The listing builds one solid part. Answer for the finished solid, in the listing's coordinates (mm). Face numbers are marked on the shaded views. A direction names the side the tool comes from. Coordinates: 2 decimals unless noted, no trailing zeros. Loops run counter-clockwise (first coordinate to the right, second up) from the corner with the lowest first, then second, coordinate; pieces in that order, holes last. Notation, with made-up numbers: M 2,-27.5 L 51,-27.5 A18 cw 51,-8.5 Z; hole C 0,-1 d6. An arc over 180 degrees is marked long. Answer as a JSON object with one key per item and string values. Group by question number.
1. A cutting plane is placed at B-B on x = -224. Give the vertices of the cut face in (y, z), and give its area (3 significant figures).
2. A cutting plane is placed at A-A on y = 261.5. Give the vertices of the cut face in (x, z).
3. Given pin 1 (9.5 mm diameter, centred on y = 180.5, z = 70.5, fed in from -X); pin 2 (6 mm diameter, centred on y = 60.5, z = 75, fed in from +X); pin 3 (7.5 mm diameter, centred on y = 110.5, z = 70.5, fed in from -X); pin 4 (9 mm diameter, centred on x = -380, z = 141.75, fed in from -Y), each flat-ended and moving along its own axis, determine where each tip first touches the part or whether it passes through.
4. For the marked faces 1 and 2, determine the directions among +Z, -Z, +X, -X, +Y, -Y from which every point of the face is accessible in a straight line to the end or side of a thin tool.
5. A cutting plane is placed at C-C on z = 91.5. Give the vertices of the cut face in (x, y).
6. Straight lines are drawn through the part: L1, parallel to Z at x = -380, y = 16; L2, parallel to X at y = 19, z = 79.25; L3, parallel to Z at x = -440, y = 180.5. For each, find the intervals that lie inside material, in ascending order.
7. A cutting plane is placed at D-D on y = 125. Give the vertices of the cut face in (x, z), and give its area (3 significant figures).
Autodesk Inventor part; units mm, degrees
ref_plane "YZ Plane" through (0, 0, 0) normal (1, 0, 0) x (0, 1, 0)
ref_plane "XZ Plane" through (0, 0, 0) normal (0, 1, 0) x (-1, 0, 0)
ref_plane "XY Plane" through (0, 0, 0) normal (0, 0, 1) x (1, 0, 0)
sketch "Sketch5" plane through (0, 0, 0) normal (0, 1, 0) x (-1, 0, 0)
  line L0 (452.5, 48) -> (452.5, 173)
  line L1 (117.5, 98) -> (117.5, 48)
  line L2 (117.5, 48) -> (452.5, 48)
  line L3 (67.5, 173) -> (67.5, 98)
  line L4 (67.5, 98) -> (117.5, 98)
  line L5 (67.5, 173) -> (452.5, 173)
  dimension "d8" = 125
  dimension "d13" = 385
  dimension "d18" = 50
  dimension "d42" = 50
extrude "Extrusion5" add sketch "Sketch5" along normal blind 291
sketch "Sketch6" plane through (0, 291, 0) normal (0, 1, 0) x (1, 0, 0)
  line L0 (-452.5, -173) -> (-67.5, -173)
  line L1 (-117.5, -48) -> (-452.5, -48)
  circle A0 centre (-140, -141.75) radius 6
  circle A1 centre (-140, -79.25) radius 6
  circle A2 centre (-260, -141.75) radius 6
  circle A3 centre (-260, -79.25) radius 6
  circle A4 centre (-380, -141.75) radius 6
  circle A5 centre (-380, -79.25) radius 6
  line L2 (-452.5, -48) -> (-452.5, -173)
  line L3 (-67.5, -173) -> (-67.5, -98)
  point P0 (0, 0)
  point P1 (-260, -173)
  dimension "d19" = 12
  dimension "d20" = 120
  dimension "d21" = 385
  dimension "d22" = 125
  dimension "d23" = 120
  dimension "d24" = 62.5
  dimension "d25" = 31.25
  dimension "d26" = 31.25
  dimension "d41" = 72.5
  dimension "d61" = 72.5
  dimension "d62" = 192.5
hole "Hole1" at (-140, 291, 141.75) at (-260, 291, 141.75) at (-380, 291, 141.75) at (-380, 291, 79.25) at (-260, 291, 79.25) at (-140, 291, 79.25) direction (0, -1, 0) diameter 10.106 depth 35 tip angle 118
sketch "Sketch7" plane through (0, 0, 0) normal (0, -1, 0) x (1, 0, 0)
  circle A0 centre (-380, 141.75) radius 5.053
  circle A1 centre (-380, 79.25) radius 5.053
  circle A2 centre (-260, 141.75) radius 5.053
  circle A3 centre (-260, 79.25) radius 5.053
  circle A4 centre (-140, 141.75) radius 5.053
  circle A5 centre (-140, 79.25) radius 5.053
  circle A6 centre (-140, 141.75) radius 5.053
  circle A7 centre (-140, 79.25) radius 5.053
  circle A8 centre (-260, 79.25) radius 5.053
  circle A9 centre (-260, 141.75) radius 5.053
  circle A10 centre (-380, 141.75) radius 5.053
  circle A11 centre (-380, 79.25) radius 5.053
  point P0 (0, 0)
hole "Hole2" at (-380, 0, 141.75) at (-380, 0, 79.25) at (-260, 0, 79.25) at (-260, 0, 141.75) at (-140, 0, 141.75) at (-140, 0, 79.25) direction (0, 1, 0) diameter 10.106 depth 35 tip angle 118
chamfer "Chamfer1" distance 5 angle 45 2 edges at (-67.5, 145.5, 98) (-117.5, 145.5, 48)
sketch "Sketch8" plane through (0, 291, 0) normal (0, 1, 0) x (1, 0, 0)
  line L0 (-182.5, -141.75) -> (-207.5, -141.75) construction
  line L1 (-182.5, -135.75) -> (-207.5, -135.75)
  line L2 (-207.5, -147.75) -> (-182.5, -147.75)
  arc A0 (-182.5, -147.75) -> (-182.5, -135.75) centre (-182.5, -141.75) ccw
  arc A1 (-207.5, -135.75) -> (-207.5, -147.75) centre (-207.5, -141.75) ccw
  line L3 (-427.5, -141.75) -> (-452.5, -141.75) construction
  line L4 (-427.5, -135.75) -> (-452.5, -135.75)
  line L5 (-452.5, -147.75) -> (-427.5, -147.75)
  arc A2 (-427.5, -147.75) -> (-427.5, -135.75) centre (-427.5, -141.75) ccw
  arc A3 (-452.5, -135.75) -> (-452.5, -147.75) centre (-452.5, -141.75) ccw
  line L6 (-452.5, -48) -> (-452.5, -173)
  circle A4 centre (-260, -141.75) radius 5.053
  point P0 (0, 0)
  point P1 (-440, -141.75)
  point P2 (-195, -141.75)
  point P3 (-440, -141.75)
  point P4 (-195, -147.75)
  point P5 (-195, -141.75)
  dimension "d46" = 12
  dimension "d47" = 12
  dimension "d48" = 25
  dimension "d49" = 25
  dimension "d58" = 12.5
  dimension "d60" = 257.5
extrude "Extrusion6" cut sketch "Sketch8" against normal blind 5 contours A0 L2 A1 L1 | A2 L5 L6 L4 | L6 A3
sketch "Sketch9" plane through (0, 0, 0) normal (0, -1, 0) x (1, 0, 0)
  line L0 (-452.5, 141.75) -> (-427.5, 141.75) construction
  line L1 (-452.5, 135.75) -> (-427.5, 135.75)
  line L2 (-427.5, 147.75) -> (-452.5, 147.75)
  arc A0 (-452.5, 147.75) -> (-452.5, 135.75) centre (-452.5, 141.75) ccw
  arc A1 (-427.5, 135.75) -> (-427.5, 147.75) centre (-427.5, 141.75) ccw
  line L3 (-207.5, 141.75) -> (-182.5, 141.75) construction
  line L4 (-207.5, 135.75) -> (-182.5, 135.75)
  line L5 (-182.5, 147.75) -> (-207.5, 147.75)
  arc A2 (-207.5, 147.75) -> (-207.5, 135.75) centre (-207.5, 141.75) ccw
  arc A3 (-182.5, 135.75) -> (-182.5, 147.75) centre (-182.5, 141.75) ccw
  arc A4 (-427.5, 135.75) -> (-427.5, 147.75) centre (-427.5, 141.75) ccw
  arc A5 (-207.5, 147.75) -> (-207.5, 135.75) centre (-207.5, 141.75) ccw
  arc A6 (-182.5, 135.75) -> (-182.5, 147.75) centre (-182.5, 141.75) ccw
  line L6 (-452.5, 48) -> (-452.5, 173)
  point P0 (0, 0)
  point P1 (-440, 141.75)
  point P2 (-195, 141.75)
  dimension "d76" = 25
  dimension "d77" = 25
  dimension "d78" = 12.5
extrude "Extrusion7" cut sketch "Sketch9" against normal blind 5
sketch "Sketch10" plane through (-452.5, 0, 48) normal (0, 0, -1) x (-1, 0, 0)
  line L0 (0, 0) -> (0, 291)
  line L1 (-330, 291) -> (0, 291)
  circle A0 centre (-295, 145.5) radius 5
  circle A1 centre (-165, 145.5) radius 5
  circle A2 centre (-35, 145.5) radius 5
  point P0 (-452.5, 0)
  point P1 (0, 145.5)
  point P2 (-165, 291)
  dimension "d63" = 130
  dimension "d64" = 130
  dimension "d65" = 10
hole "Hole3" at (-157.5, 145.5, 48) at (-287.5, 145.5, 48) at (-417.5, 145.5, 48) direction (0, 0, 1) diameter 8.376 depth 25 tip angle 118
chamfer "Chamfer2" distance 0.5 angle 45 14 edges at (-195, 291, 147.75) (-213.5, 291, 141.75) (-195, 291, 135.75) (-176.5, 291, 141.75) (-440, 291, 147.75) (-440, 291, 135.75) (-421.5, 291, 141.75) (-213.5, 0, 141.75) (-195, 0, 147.75) (-176.5, 0, 141.75) (-195, 0, 135.75) (-440, 0, 147.75) (-421.5, 0, 141.75) (-440, 0, 135.75)
chamfer "Chamfer3" distance 2 angle 45 3 edges at (-67.5, 145.5, 173) (-452.5, 145.5, 173) (-452.5, 145.5, 48)
sketch "Sketch11" plane through (-450.5, 0, 173) normal (0, 0, 1) x (1, 0, 0)
  circle A0 centre (226.5, 145.5) radius 7.5
  line L0 (-2, 291) -> (-2, 0)
  point P0 (450.5, 0)
  point P1 (-2, 145.5)
  dimension "d82" = 228.5
  dimension "d83" = 15
hole "Hole4" at (-224, 145.5, 173) direction (0, 0, -1) diameter 15 end through all
sketch "Sketch12" plane through (-452.5, 286, 135.75) normal (-1, 0, 0) x (0, 0, 1)
  line L0 (-85.75, -286) -> (-85.75, 5)
  line L1 (-85.75, -286) -> (-0.5, -286)
  line L2 (-85.75, 5) -> (-0.5, 5)
  circle A0 centre (-65.25, -105.5) radius 5
  circle A1 centre (14.75, -105.5) radius 5
  circle A2 centre (-65.25, -175.5) radius 5
  circle A3 centre (14.75, -175.5) radius 5
  line L3 (-85.75, -140.5) -> (-93.0771, -140.5)
  line L4 (37.25, -286) -> (37.25, 5)
  line L5 (-87.75, 5) -> (-87.75, -286)
  point P0 (-135.75, -286)
  dimension "d91" = 10
  dimension "d92" = 80
  dimension "d94" = 70
  dimension "d96" = 35
  dimension "d97" = 125
  dimension "d99" = 22.5
  dimension "d100" = 110.5
  dimension "d101" = 110.5
hole "Hole5" at (-452.5, 180.5, 150.5) at (-452.5, 180.5, 70.5) at (-452.5, 110.5, 150.5) at (-452.5, 110.5, 70.5) direction (1, 0, 0) diameter 8.376 depth 25 tip angle 118
equation "\"d20\" = d23"
equation "\"d25\" = -0.5 * d24 + 0.5 * d22"
equation "\"d47\" = d46"
equation "\"d49\" = d48"
equation "\"d64\" = d63"
equation "\"d96\" = 0.5 * d94"
equation "\"d99\" = -0.5 * d92 + 0.5 * d97"
properties part number "BC-10010" material "Alumínio 7075"
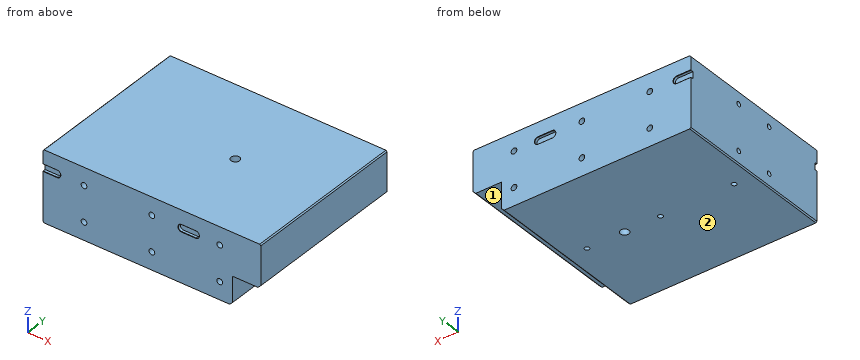
From the geometry:
{
 "1": {"outline": "M 0,48 L 138,48 L 138,173 L 0,173 Z; M 153,48 L 291,48 L 291,173 L 153,173 Z", "area": "34,500 mm²"},
 "2": {"outline": "M -452.5,50 L -450.5,48 L -122.5,48 L -117.5,53 L -117.5,98 L -72.5,98 L -67.5,103 L -67.5,171 L -69.5,173 L -450.5,173 L -452.5,171 Z; hole C -380,79.25 d10.11; hole C -380,141.75 d10.11; hole C -260,79.25 d10.11; hole C -260,141.75 d10.11; hole C -140,79.25 d10.11; hole C -140,141.75 d10.11"},
 "3": {"pin 1": "stops at x = -452.5", "pin 2": "stops at x = -117.5", "pin 3": "stops at x = -427.24", "pin 4": "stops at y = 35.33"},
 "4": {"face 1": "-Z, +X, +Y, -Y", "face 2": "-Z, +X, -X, +Y, -Y"},
 "5": {"outline": "M -452.5,0 L -117.5,0 L -117.5,291 L -452.5,291 Z; hole C -224,145.5 d15"},
 "6": {"L1": "z = 48 to 74.2, 84.3 to 136.7, 146.8 to 173", "L2": "x = -452.5 to -385.05, -374.95 to -265.05, -254.95 to -145.05, -134.95 to -117.5", "L3": "z = 48 to 66.31, 74.69 to 146.31, 154.69 to 173"},
 "7": {"outline": "M -452.5,50 L -450.5,48 L -122.5,48 L -117.5,53 L -117.5,98 L -72.5,98 L -67.5,103 L -67.5,171 L -69.5,173 L -450.5,173 L -452.5,171 Z", "area": "45,600 mm²"}
}
